```python
from build123d import *

# Parameters (mm, degrees)
SKETCH2_W          = 278.036516336
SKETCH2_H          = 207.466179174
CUT_EXTRUDE1_DEPTH = 413.310562562


with BuildPart() as part:
    # Sketch1 → Revolve1 (revolve)
    with BuildSketch(Plane.XY, mode=Mode.PRIVATE) as revolve1_sk:
        Polygon((-30, 150), (-80, 150), (-80, 100), (-140, 100), (-140, 50), (-200, 50), (-200, -70), (-80, -70), (-80, -150), (-40, -150), (-40, -30), (-140, -30), (-140, 30), (-80, 30), (-80, 80), (-50, 80), (-50, 130), (-30, 130), align=None)
    revolve(revolve1_sk.sketch.rotate(Axis((0, -150, 0), (0, 1, 0)), 270), axis=Axis((0, -150, 0), (0, 1, 0)))

    # Sketch2 → Cut-Extrude1 (cut, through all)
    with BuildSketch(Plane(origin=(0, 150, 0), x_dir=(1, 0, 0), z_dir=(0, 1, 0))):
        with Locations((-139.018258168, 103.733089587)):
            Rectangle(SKETCH2_W, SKETCH2_H)
    extrude(amount=-CUT_EXTRUDE1_DEPTH, mode=Mode.SUBTRACT)


solid = part.part
```
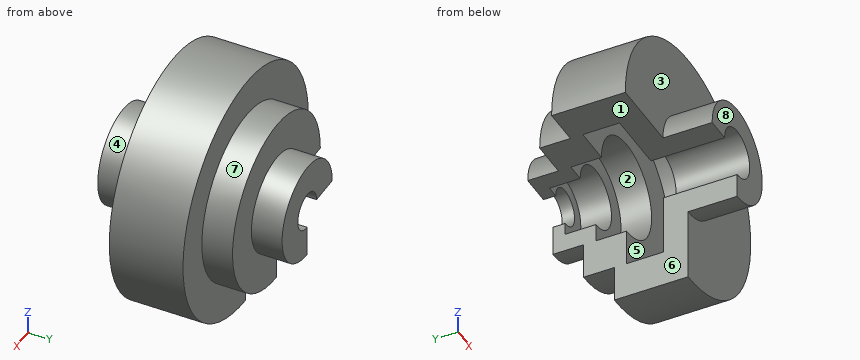
Input: part model. Units: mm. Frame: model coordinates. Face numbers are marked on the shaded views. A direction names the side the tool comes from. Coordinates: 2 decimals unless noted, no trailing zeros. Loops run counter-clockwise (first coordinate to the right, second up) from the corner with the lowest first, then second, coordinate; pieces in that order, holes last. Notation, with made-up numbers: M 85.25,60.25 L 130.25,60.25 A22 ccw 130.25,94.25 Z; hole C 22,57.25 d5. An arc over 180 degrees is marked long. Use a Markdown table: item, result. Add a question column.
1) Line query: L1, parallel to Y at x = 76, z = 14.5; L2, parallel to Y at x = 80, z = 20.5; L3, parallel to Y at x = -129, z = 106. Output: solid intervals per line, ascending. Write a range as from..to.
2) Section A-A, the plane x = 112.5. Return the cut outline in (y, z).
3) Set-up query: the marked faces 4, 5, 6, 7 and 8. Return all of +Z, -Z, +X, -X, +Y, -Y with unobstructed straight access to the full face (end or side cutting, diameter ignored); none if empty.
4) Section B-B, the plane z = -114. Return the cut outline in (x, y) (3 decimals).
5) Draft query along Z for the marked faces 1, 2 and 3. Return one class per face: +Z half, -Z half, draft (parallel to the pull), parting line (faces both ways), or undercut.
6) Pin query (flat end, axial travel): P1, Ø2, axis at x = -78, z = 134, coming from the +Y side; P2, Ø1.5, axis at x = -43.5, y = -98.5, coming from the +Z side; P3, Ø3, axis at x = 113, z = 7.5, coming from the -Y side. Return the tip coordinate at first contact, or that it passes through.
7) Section D-D, the plane x = -125.5. Return the cut outline in (y, z), plus the area to 3 significant figures.
8) Section C-C, the plane y = 7. Return the cut outline in (x, z), plus the area to 3 significant figures.
Answer below:
| question | item | result |
|---|---|---|
| 1 | L1 | -150..-30, 80..150 |
| 1 | L2 | -70..-30, 30..100 |
| 1 | L3 | -70..50 |
| 2 | outline | M -70,-165.36 L 50,-165.36 L 50,-83.33 L 100,-83.33 L 100,83.33 L 50,83.33 L 50,165.36 L -70,165.36 Z; hole M -30,-83.33 L 30,-83.33 L 30,83.33 L -30,83.33 Z |
| 3 | face 4 | -Y |
| 3 | face 5 | none |
| 3 | face 6 | -Z, -X, +Y, -Y |
| 3 | face 7 | +Y |
| 3 | face 8 | +Z, -Z, +X, -X, -Y |
| 4 | outline | M 0,-70 L 164.329,-70 L 164.329,50 L 81.265,50 L 81.265,100 L 0,100 L 0,30 L 81.265,30 L 81.265,-30 L 0,-30 Z |
| 5 | face 1 | -Z half |
| 5 | face 2 | undercut |
| 5 | face 3 | draft |
| 6 | P1 | y = 50 |
| 6 | P2 | z = 67.62 |
| 6 | P3 | y = -70 |
| 7 | outline | M -70,0 L -30,0 L -30,62.05 L 30,62.05 L 30,0 L 100,0 L 100,62.05 L 50,62.05 L 50,155.72 L -70,155.72 Z |
| 7 | area | 18,100 mm2 |
| 8 | outline | M -200,0 L -140,0 A140 cw long 0,-140 L 0,-200 A200 ccw long Z |
| 8 | area | 48,100 mm2 |
